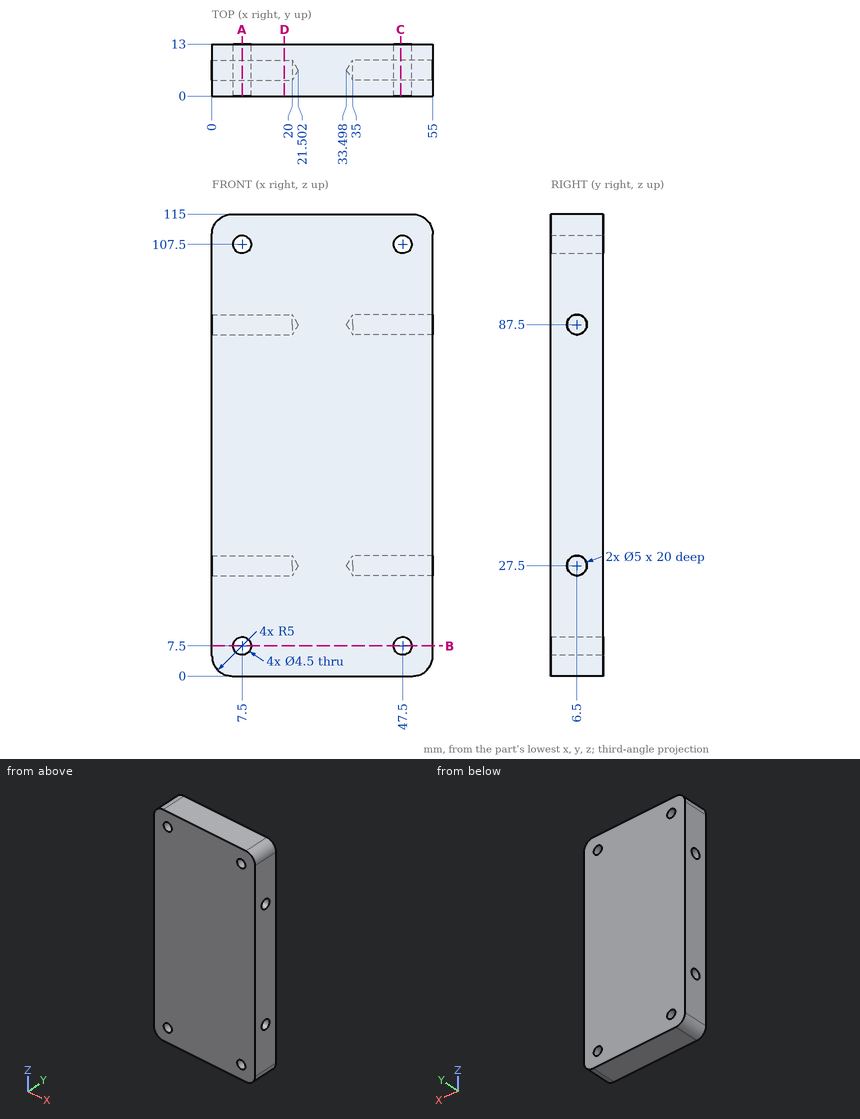
Geometry: see drawing. Coordinates: mm, zero at the bounding-box minimum. Round coordinates to 2 decimals unless told otherwise and drop trailing zeros. Order: outer loops, then holes, each group sorted by start corner. A loop starts at its lowest first (then second) coordinate and runs counter-clockwise, first axis right, second up. Notation, with made-up numbers: (-30.75, 15.25) - (9.25, 15.25) arc R26 ccw to (9.25, 51.25) - close; hole circle Ø6 at (-32.75, 42). An arc over 180 degrees is marked (long way). One line per question, with ' | ' between items. Start each with the question number.
1) Cut plane A-A, the plane x = 7.5. Return the cut outline in (y, z), then the cut area to 3 significant figures.
2) Cut plane C-C, the plane x = 47. Return the cut outline in (y, z).
3) Cut plane B-B, the plane z = 7.5. Return the cut outline in (x, y).
4) Ray query, probe 1 along Z at (x, y) = (7.5, 9.75); probe 2 along Z at (x, y) = (8, 6.5); probe 3 along Z at (x, y) = (15.5, 6.25). Return the intervals inside material, ascending.
5) Contact query for flat-ended pins moving along their axis: P1, Ø3.5, axis at x = 7.5, z = 7.5, coming from the -Y side; P2, Ø4.5, axis at y = 6.5, z = 87.5, coming from the +X side; P3, Ø4.5, axis at y = 6.5, z = 27.5, coming from the -X side. Output: stop coordinate, or through.
6) Cut plane D-D, the plane x = 18. Return the cut outline in (y, z).
Worked out:
1) outline: (0, 0) - (13, 0) - (13, 5.25) - (0, 5.25) - close; (0, 9.75) - (13, 9.75) - (13, 105.25) - (0, 105.25) - close; (0, 109.75) - (13, 109.75) - (13, 115) - (0, 115) - close; hole circle Ø5 at (6.5, 27.5); hole circle Ø5 at (6.5, 87.5) | area: 1,340 mm^2
2) outline: (0, 0) - (13, 0) - (13, 5.31) - (0, 5.31) - close; (0, 9.69) - (13, 9.69) - (13, 105.31) - (0, 105.31) - close; (0, 109.69) - (13, 109.69) - (13, 115) - (0, 115) - close; hole circle Ø5 at (6.5, 27.5); hole circle Ø5 at (6.5, 87.5)
3) outline: (0, 0) - (5.25, 0) - (5.25, 13) - (0, 13) - close; (9.75, 0) - (45.25, 0) - (45.25, 13) - (9.75, 13) - close; (49.75, 0) - (55, 0) - (55, 13) - (49.75, 13) - close
4) probe 1: z = 0 to 5.25, 9.75 to 105.25, 109.75 to 115 | probe 2: z = 0 to 5.31, 9.69 to 25, 30 to 85, 90 to 105.31, 109.69 to 115 | probe 3: z = 0 to 25.01, 29.99 to 85.01, 89.99 to 115
5) P1: passes through | P2: stops at x = 34.85 | P3: stops at x = 20.15
6) outline: (0, 0) - (13, 0) - (13, 115) - (0, 115) - close; hole circle Ø5 at (6.5, 27.5); hole circle Ø5 at (6.5, 87.5)
